```python
from build123d import *

# Parameters (mm, degrees)
F0_W         = 50.8
F0_H         = 44.45
F1_DEPTH     = 38.1
F2_W         = 13.97
F2_H         = 5.08
F3_DEPTH     = 50.8
F4_R         = 12.7
F5_W         = 45.72
F5_H         = 13.97
F6_DEPTH     = 50.8
F7_R         = 5.08
F8_W         = 14.097
F8_H         = 15.24
F9_DEPTH     = 50.8
F10_R        = 5.07999
F11_T        = 2.54
F11_T3_DEPTH = 9.0721543583
F11_T5_DEPTH = 9.0721543583
F11_T7_DEPTH = 9.144
F11_T9_DEPTH = 9.144


# Not quite as in the source:
# - a fillet or chamfer is up to 0.001 mm smaller than in the source, because OpenCascade refuses the exact size
# - a shell that OpenCascade refuses in one call is made with other operations: the cavity is built on its own and cut out


with BuildPart() as f1:
    # F0 (on Top) → F1 (new body)
    with BuildSketch(Plane.XY):
        Rectangle(F0_W, F0_H)
    extrude(amount=F1_DEPTH)

    # F2 (on face) → F3 (cut)
    with BuildSketch(Plane.YZ.offset(25.4)):
        with Locations((15.24, 2.54)):
            Rectangle(F2_W, F2_H)
    extrude(amount=-F3_DEPTH, mode=Mode.SUBTRACT)

    # F4
    f4_edges = [f1.edges().sort_by_distance(p)[0] for p in [
        (0, 22.225, 38.1),
    ]]
    fillet(f4_edges, radius=F4_R)

    # F5 (on face) → F6 (cut)
    with BuildSketch(Plane(origin=(0, 22.225, 0), x_dir=(-1, 0, 0), z_dir=(0, 1, 0))):
        with Locations((0, 28.575)):
            Rectangle(F5_W, F5_H)
    extrude(amount=-F6_DEPTH, mode=Mode.SUBTRACT)

    # F7
    f7_edges = [f1.edges().sort_by_distance(p)[0] for p in [
        (22.86, -2.54, 35.56),
        (-22.86, -2.54, 35.56),
    ]]
    fillet(f7_edges, radius=F7_R)

    # F8 (on face) → F9 (cut)
    with BuildSketch(Plane.YZ.offset(25.4)):
        with BuildLine():
            ThreePointArc((18.161, 26.3400295448), (18.1977232283, 26.7491865029), (18.2099788483, 27.1598053184))
            ThreePointArc((18.2099788483, 27.1598053184), (18.1977232283, 27.5704241338), (18.161, 27.9795810919))
            Line((18.161, 27.9795810919), (18.161, 26.3400295448))
        make_face()
        with BuildLine():
            Line((18.161, 26.3400295448), (18.161, 27.9795810919))
            ThreePointArc((18.161, 27.9795810919), (15.7632997742, 32.4232792644), (10.978474631, 34.036))
            ThreePointArc((10.978474631, 34.036), (6.2916716696, 22.46222933), (18.161, 26.3400295448))
        make_face()
        with BuildLine():
            Line((18.161, 18.796), (18.161, 26.3400295448))
            ThreePointArc((18.161, 26.3400295448), (6.2916716696, 22.46222933), (10.978474631, 34.036))
            Line((10.978474631, 34.036), (0, 34.036))
            Line((0, 34.036), (0, 18.796))
            Line((0, 18.796), (18.161, 18.796))
        make_face()
        with Locations((-11.1125, 26.416)):
            Rectangle(F8_W, F8_H)
    extrude(amount=-F9_DEPTH, mode=Mode.SUBTRACT)

    # F10 (radius 5.08 in the source; OpenCascade refuses exactly that, so slightly less here)
    f10_edges = [f1.edges().sort_by_distance(p)[0] for p in [
        (0, 8.255, 5.08),
    ]]
    fillet(f10_edges, radius=F10_R)

    # F11: shell of thickness 2.54, made by hand


with BuildPart() as f11_core1:
    # F11_t2: copy of F1
    add(f1.part)

    # the walls: a layer under each face that stays
    f11_faces = [f11_core1.faces().sort_by_distance(p)[0] for p in [
        (-25.4, 14.8166666667, 6.35),
        (0, 17.779995, 5.08),
        (0, 9.7428946226, 3.5921053774),
        (0, 22.225, 15.24),
        (0, 8.255, 5e-06),
        (16.9333333333, 12.8120018728, 37.6672579939),
        (0, -6.985, 0),
        (0, -6.35, 38.1),
        (0, -22.225, 19.05),
        (-23.4039228208, 5.4892373155, 34.036),
        (-23.3996024836, 16.3584390419, 31.8573813067),
        (-23.4039228208, -11.1125, 34.036),
        (-16.9333333333, -18.161, 21.336),
        (25.4, -14.8166666667, 6.35),
        (-22.86, 19.7907563947, 26.035),
        (0, 20.193, 21.59),
        (22.86, 19.7907563947, 26.035),
        (-21.3721024484, -0.5301288674, 34.0721024484),
        (0, -2.54, 35.56),
        (21.3721024484, -0.5301288674, 34.0721024484),
        (22.86, -20.193, 26.035),
        (0, -20.193, 21.59),
        (-22.86, -20.193, 26.035),
        (-22.86, -2.032, 26.035),
        (22.86, -2.032, 26.035),
        (23.4039228208, 5.4892373155, 34.036),
        (23.3996024836, 16.3584390419, 31.8573813067),
        (23.4039228208, -11.1125, 34.036),
    ]]
    thicken(f11_faces, amount=-F11_T, mode=Mode.SUBTRACT)

    # F11_s4 → F11_t3 (cut)
    with BuildSketch(Plane.YZ.offset(-27.94)):
        Polygon((-18.1356, 34.0106), (-18.161, 36.576), (-20.701, 36.576), (-20.701, 34.036), align=None)
    extrude(amount=F11_T3_DEPTH, mode=Mode.SUBTRACT)

    # F11_s6 → F11_t5 (cut)
    with BuildSketch(Plane.YZ.offset(18.8678456417)):
        Polygon((-18.1356, 34.0106), (-20.701, 34.036), (-20.701, 36.576), (-18.161, 36.576), align=None)
    extrude(amount=F11_T5_DEPTH, mode=Mode.SUBTRACT)

    # F11_s8 → F11_t7 (cut)
    with BuildSketch(Plane.XZ.offset(-24.765)):
        Polygon((-22.8346, 21.6154), (-25.4, 21.59), (-25.4, 19.05), (-22.86, 19.05), align=None)
        Polygon((22.8346, 21.6154), (22.86, 19.05), (25.4, 19.05), (25.4, 21.59), align=None)
    extrude(amount=F11_T7_DEPTH, mode=Mode.SUBTRACT)

    # F11_s10 → F11_t9 (cut)
    with BuildSketch(Plane.XZ.offset(15.621)):
        Polygon((22.8346, 21.6154), (25.4, 21.59), (25.4, 19.05), (22.86, 19.05), align=None)
        Polygon((-22.8346, 21.6154), (-22.86, 19.05), (-25.4, 19.05), (-25.4, 21.59), align=None)
    extrude(amount=F11_T9_DEPTH, mode=Mode.SUBTRACT)


with BuildPart() as f1_1:
    add(f1.part)

    # what is left inside the walls is the cavity
    f11_cavity = [f11_core1.part.solids().sort_by_distance(p)[0] for p in [
        (0, -11.073069, 2.5654),
    ]]
    add(f11_cavity, mode=Mode.SUBTRACT)


solid = f1_1.part
```
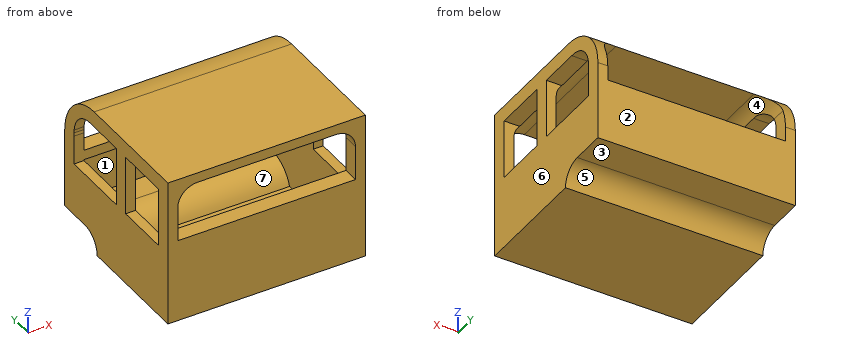
For this review, take the finished solid that the model builds, in its own axes (mm). Face numbers are marked on the shaded views. A direction names the side the tool comes from. Coordinates: 2 decimals unless noted, no trailing zeros. Write each loop counter-clockwise with the first axis right and the second up, starting at its lowest first coordinate (ties: lowest second). Pieces come first, ordered by that corner, then holes.
(1) Add section D-D on z = 32.5. Give the boundary of the cut face in (x, y) (3 decimals), then the cut area to 3 significant figures.
(2) Tool access review of the marked faces 1, 2, 3 and 4: name each direction out of +Z, -Z, +X, -X, +Y, -Y from which nothing blocks a thin tool from reaching the whole face with its end or side.
(3) For pin 1 Ø1.2 at (x, y) = (-2.5, 20) entering from +Z; pin 2 Ø3 at (x, y) = (-23.5, 13.5) entering from +Z; pin 3 Ø12 at (x, y) = (4, 17.5) entering from -Z, all flat-tipped, find the tip position at first contact; note any pin that passes through.
(4) The part is to be moulded in two halves that separate along Y. For the marked faces 5, 6 and 7, say which applies: +Y half, -Y half, draft (parallel to the pull), parting line (faces both ways), or undercut.
(5) Add section C-C on z = 16. Give the boundary of the cut face in (x, y) (3 decimals), then the cut area to 3 significant figures.
(6) Add section A-A on y = -12. Give the boundary of the cut face in (x, z), then the cut area to 3 significant figures.
(7) Wall thickness on probe 1 along Z at (x, y) = (-9, 1.5); probe 2 along X at (y, z) = (-10, 7.5); probe 3 along Y at (x, z) = (-11, 10) (3 decimals): over which ranges is each line inside the solid? List them lowest first.
Answer sheet:
1. outline: (-25.4, -22.225) - (-22.441, -22.225) - (-22.441, -18.161) - (-25.4, -18.161) - close; (-25.4, -4.064) - (-22.441, -4.064) - (-22.441, 0) - (-25.4, 0) - close; (-25.4, 15.671) - (-22.441, 15.671) - (-22.441, 20.055) - (-25.4, 20.055) - close; (22.441, -22.225) - (25.4, -22.225) - (25.4, -18.161) - (22.441, -18.161) - close; (22.441, -4.064) - (25.4, -4.064) - (25.4, 0) - (22.441, 0) - close; (22.441, 15.671) - (25.4, 15.671) - (25.4, 20.055) - (22.441, 20.055) - close
1. area: 74.0 mm2
2. face 1: none
2. face 2: +Z, -Z, +X, -X, +Y
2. face 3: -Z, +X, -X, +Y
2. face 4: +Y, -Y
3. pin 1: stops at z = 21.59
3. pin 2: stops at z = 37.86
3. pin 3: stops at z = 4.74
4. face 5: +Y half
4. face 6: draft
4. face 7: undercut
5. outline: (-25.4, -22.225) - (25.4, -22.225) - (25.4, 22.225) - (-25.4, 22.225) - close; hole (-22.86, -19.685) - (22.86, -19.685) - (22.86, 19.685) - (-22.86, 19.685) - close
5. area: 458 mm2
6. outline: (-25.4, 0) - (25.4, 0) - (25.4, 18.8) - (22.86, 18.8) - (22.86, 2.54) - (-22.86, 2.54) - (-22.86, 18.8) - (-25.4, 18.8) - close; (-25.4, 34.04) - (-21.41, 34.04) arc R5.08 cw to (-17.78, 35.56) - (17.78, 35.56) arc R5.08 cw to (21.41, 34.04) - (25.4, 34.04) - (25.4, 38.1) - (-25.4, 38.1) - close
6. area: 356 mm2
7. probe 1: z = 0 to 2.54, 35.56 to 38.1
7. probe 2: x = -25.4 to -22.86, 22.86 to 25.4
7. probe 3: y = -22.225 to -19.685, 19.685 to 22.225
